Could you check a few things on this model? Use its own coordinates, in mm. Face numbers are marked on the shaded views. A direction names the side the tool comes from. Give positions to 0.01 mm unless a question says otherwise; leave off trailing zeros. Loops run counter-clockwise (first coordinate to the right, second up) from the corner with the lowest first, then second, coordinate; pieces in that order, holes last. Notation, with made-up numbers: (24, 31) -> (80, 31) arc R30 cw to (80, 64) -> close; hole circle Ø11 at (82.5, 78). An arc over 180 degrees is marked (long way). Put each result on its own line as item: value.
```python
from build123d import *

# Parameters (mm, degrees)
BOSS_EXTRUDE1_DEPTH = 11.5
BOSS_EXTRUDE2_DEPTH = 3.5
SKETCH4_R           = 1.5
BOSS_EXTRUDE3_DEPTH = 3
SKETCH5_R           = 1.25
CUT_EXTRUDE1_DEPTH  = 3.5


with BuildPart() as part:
    # Sketch1 → Boss-Extrude1 (new body)
    with BuildSketch(Plane(origin=(0, 0, 0), x_dir=(1, 0, 0), z_dir=(0, 1, 0))):
        Polygon((-20, 0), (-24, 0), (-24, 22), (-20, 22), (-20, 26), (-18, 26), (-18, 22), (0, 22), (0, 0), (-18, 0), (-18, -4), (-20, -4), align=None)
    extrude(amount=BOSS_EXTRUDE1_DEPTH)

    # Sketch2 → Boss-Extrude2 (add)
    with BuildSketch(Plane.ZY.offset(24)):
        with BuildLine():
            ThreePointArc((-11.140964663, 3.75), (0, 5.75), (-11.140964663, 7.75))
            ThreePointArc((-11.140964663, 7.75), (-13.140964663, 5.75), (-11.140964663, 3.75))
        make_face()
    extrude(amount=BOSS_EXTRUDE2_DEPTH)

    # Sketch4 → Boss-Extrude3 (add)
    with BuildSketch(Plane.ZY.offset(27.5)):
        with Locations((-5.75, 5.75)):
            Circle(SKETCH4_R)
    extrude(amount=BOSS_EXTRUDE3_DEPTH)

    # Sketch5 → Cut-Extrude1 (cut)
    with BuildSketch(Plane.ZY.offset(20)):
        with Locations((-24.8, 5.75)):
            Circle(SKETCH5_R)
        with Locations((2.8, 5.75)):
            Circle(SKETCH5_R)
    extrude(amount=-CUT_EXTRUDE1_DEPTH, mode=Mode.SUBTRACT)


solid = part.part
```
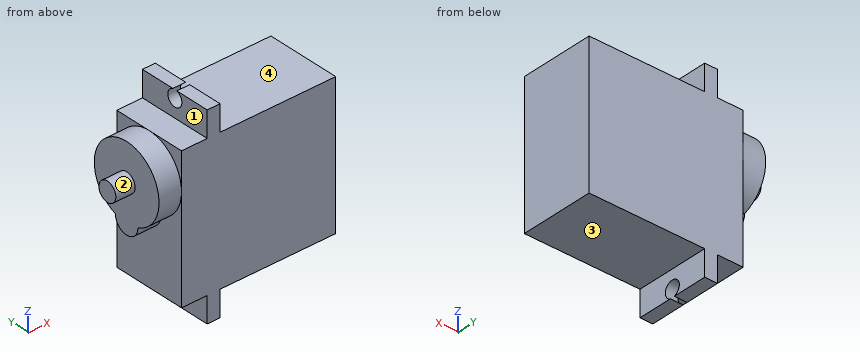
1. If we section it at D-D (y = 10.25): List the corners of the cut face in (x, z) for me.
Recorded:
outline: (-27.5, -9.33) -> (-24, -9.33) -> (-24, -22) -> (-20, -22) -> (-20, -26) -> (-18, -26) -> (-18, -22) -> (0, -22) -> (0, 0) -> (-18, 0) -> (-18, 4) -> (-20, 4) -> (-20, 0) -> (-24, 0) -> (-24, -2.17) -> (-27.5, -2.17) -> close
2. I need wall thicknesses on line 1 (Y direction, x = -19.5, z = -24.8); line 2 (Z direction, x = -13, y = 7.75); line 3 (X direction, y = 2.75, z = -12). Which ranges of each line are inside material? Lowest first, please.
Recorded:
line 1: y = 0 to 4.5, 7 to 11.5
line 2: z = -22 to 0
line 3: x = -24 to 0
3. For the marked faces 1, 2, 3 and 4, which set-ups out of +Z, -Z, +X, -X, +Y, -Y let a thin tool reach every point of the face, with its end or its side?
Recorded:
face 1: +Z, -X, +Y, -Y
face 2: -X
face 3: -Z, +X, +Y, -Y
face 4: +Z, +X, +Y, -Y
4. If we section it at B-B (z = -10.5): List the corners of the cut face in (x, y) for me.
Recorded:
outline: (-27.5, 2.51) -> (-24, 2.51) -> (-24, 0) -> (0, 0) -> (0, 11.5) -> (-24, 11.5) -> (-24, 8.99) -> (-27.5, 8.99) -> close
5. I'm going to push flat-ended pins straight in: pin 1 (1.2 mm diameter, centred on x = -21.5, y = 7, fed in from -Z); pin 2 (6.5 mm diameter, centred on y = 9.5, z = -2.5, fed in from -X); pin 3 (4.5 mm diameter, centred on y = 6.5, z = -24.5, fed in from +X). Where does each tip first touch, or does it pass through?
Recorded:
pin 1: stops at z = -22
pin 2: stops at x = -27.5
pin 3: stops at x = -18
6. If we section it at C-C (x = -2): List the corners of the cut face in (y, z) for me.
Recorded:
outline: (0, -22) -> (11.5, -22) -> (11.5, 0) -> (0, 0) -> close
7. If we section it at A-A (z = -24.8): List the corners of the cut face in (x, y) for me.
Recorded:
outline: (-20, 0) -> (-18, 0) -> (-18, 4.5) -> (-20, 4.5) -> close; (-20, 7) -> (-18, 7) -> (-18, 11.5) -> (-20, 11.5) -> close
